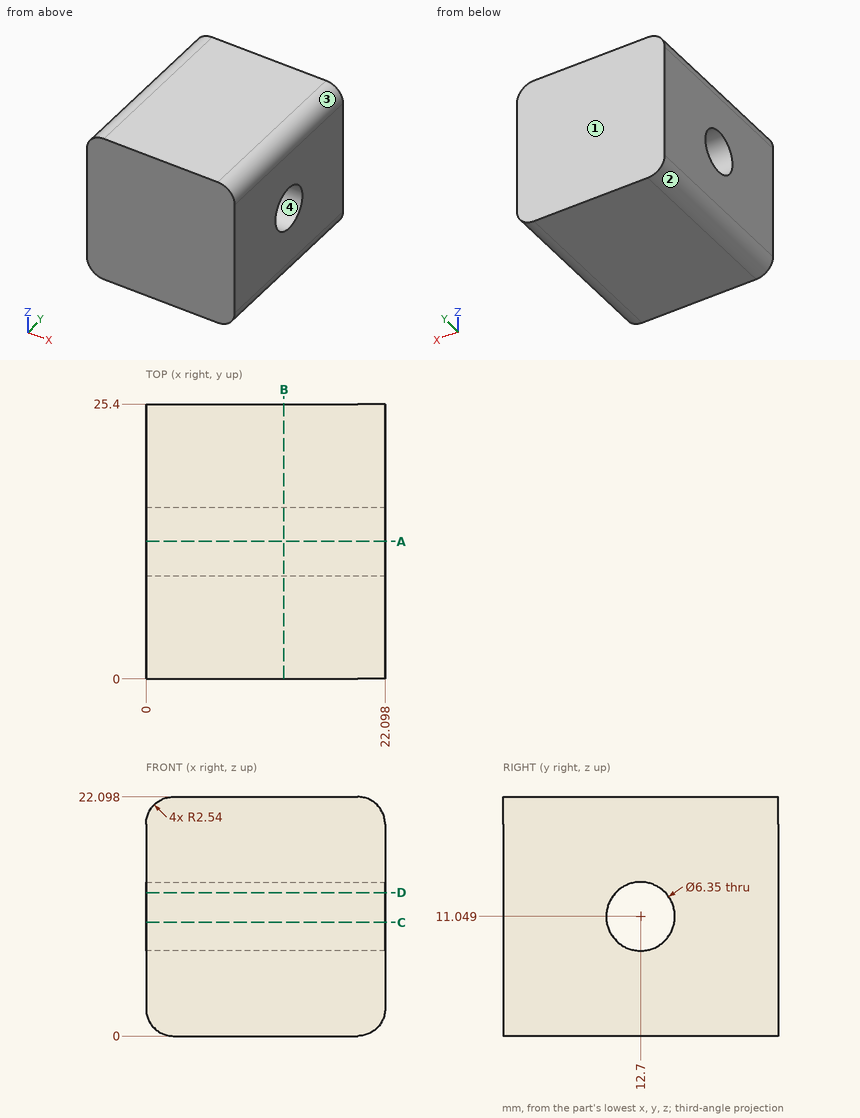
Source: three-view drawing plus pictorial views. Frame: mm from the lowest corner of the part. Round coordinates to 2 decimals unless told otherwise and drop trailing zeros. Write each loop counter-clockwise with the first axis right and the second up, starting at its lowest first coordinate (ties: lowest second). Pieces come first, ordered by that corner, then holes. Notation, with made-up numbers: M -7.5,72 L 39.5,72 A24 ccw 39.5,91 Z; hole C 76.5,-21 d2. An arc over 180 degrees is marked long. One line per item, written item: value. Start each with the question number.
Item 1: Section query C-C (z = 10.5). Return the cut outline in (x, y).
Item 2: Section query A-A (y = 12.7). Return the cut outline in (x, z).
Item 3: Mould query, pull axis Z, two halves, no side actions, for the marked faces 1, 2, 3 and 4. Classes: pulls with the +Z half, pulls with the -Z half, needs draft (parallel to the pull), parting line crosses it, or undercut.
Item 4: Section query B-B (x = 12.75). Return the cut outline in (y, z) (3 decimals), plus the area to 3 significant figures.
Item 5: Ray query, L1, parallel to Y at x = 20, z = 9; L2, parallel to Z at x = 11.5, y = 13.25; L3, parallel to Y at x = 8.25, z = 9.5. Return the intervals inside material, ascending. Write a range as from..to.
Item 6: Section query D-D (z = 13.25). Return the cut outline in (x, y).
Result set:
1. outline: M 0,0 L 22.1,0 L 22.1,9.57 L 0,9.57 Z; M 0,15.83 L 22.1,15.83 L 22.1,25.4 L 0,25.4 Z
2. outline: M 0,2.54 A2.54 ccw 2.54,0 L 19.56,0 A2.54 ccw 22.1,2.54 L 22.1,7.87 L 0,7.87 Z; M 0,14.22 L 22.1,14.22 L 22.1,19.56 A2.54 ccw 19.56,22.1 L 2.54,22.1 A2.54 ccw 0,19.56 Z
3. face 1: needs draft
3. face 2: pulls with the -Z half
3. face 3: pulls with the +Z half
3. face 4: undercut
4. outline: M 0,0 L 25.4,0 L 25.4,22.098 L 0,22.098 Z; hole C 12.7,11.049 d6.35
4. area: 530 mm²
5. L1: y = 0..10.27, 15.13..25.4
5. L2: z = 0..7.92, 14.18..22.1
5. L3: y = 0..9.93, 15.47..25.4
6. outline: M 0,0 L 22.1,0 L 22.1,10.41 L 0,10.41 Z; M 0,14.99 L 22.1,14.99 L 22.1,25.4 L 0,25.4 Z
